Here's how the part is built. I have some questions about the finished solid (model axes, mm). Face numbers are marked on the shaded views. A direction names the side the tool comes from. Coordinates: 2 decimals unless noted, no trailing zeros. Write each loop counter-clockwise with the first axis right and the second up, starting at its lowest first coordinate (ties: lowest second). Pieces come first, ordered by that corner, then holes. Notation, with made-up numbers: (71, 36) -> (116, 36) arc R22 ccw to (116, 64) -> close; hole circle Ø6 at (-9, 43.5). An arc over 180 degrees is marked (long way). Use a Markdown table: item, result. Add a question column.
Item 1: Will these pins go through, and if not, where does the flat tip stop? pin 1 Ø2.5 at (x, y) = (-2.865, 8.89) entering from +Z; pin 2 Ø2 at (x, y) = (-5.5, -9) entering from -Z (3 decimals).
Item 2: On a 3-axis mill with a long thin cutter (end or side, diameter ignored), from which of +Z, -Z, +X, -X, +Y, -Y can I reach the whole of each face in a straight line? I mean the marked faces 4, 5 and 6. Say none if no direction works.
Item 3: If I drill on line 1 along X through (y, z) = (-9, 2.75); line 2 along Y through (x, z) = (3, 6); line 3 along X through (y, z) = (-9.5, 0.5), over which ranges is the centre line in solid material (lowest first)? Write a range as from..to.
Item 4: Imagine slicing it at B-B, the plane z = 1.75. Write out the boundary of the cut face in (x, y) (3 decimals).
Item 5: Imagine slicing it at C-C, the plane x = -7. Write out the boundary of the cut face in (y, z) (3 decimals).
Item 6: Imagine slicing it at A-A, the plane y = -8.89. Write out the boundary of the cut face in (x, z) (3 decimals), and give its area (3 significant figures).
Item 7: Imagine slicing it at D-D, the plane x = -4. Write out the boundary of the cut face in (y, z).
Item 8: If we mould it in two halves opening along Y, with no side actions, what happens to the marked faces 1, 2 and 3? For each: pulls with the +Y half, pulls with the -Y half, needs draft (parallel to the pull), parting line crosses it, or undercut.
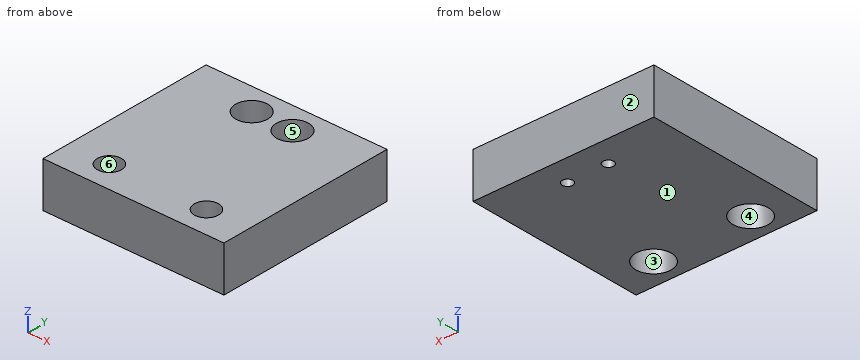
```python
from build123d import *

# Parameters (mm, degrees)
F0_W     = 25.4
F0_H     = 25.4
F0_R     = 1.7
F0_R_2   = 0.75
F1_DEPTH = 6.35
F2_R     = 2.5
F3_DEPTH = 3.175
F4_R     = 2.25
F5_DEPTH = 3.75


# Not quite as in the source:
# - a feature names something its author has since deleted; it is built from what else it names


with BuildPart() as f1:
    # F0 (on Top) → F1 (new body)
    with BuildSketch(Plane.XY):
        Rectangle(F0_W, F0_H)
        with Locations((-6.8136113696, -8.89)):
            Circle(F0_R, mode=Mode.SUBTRACT)
        with Locations((6.8136113696, -8.89)):
            Circle(F0_R, mode=Mode.SUBTRACT)
        with Locations((-2.865, 8.89)):
            Circle(F0_R_2, mode=Mode.SUBTRACT)
        with Locations((2.865, 8.89)):
            Circle(F0_R_2, mode=Mode.SUBTRACT)
    extrude(amount=F1_DEPTH)

    # F2 (on Top) → F3 (cut)
    with BuildSketch(Plane.XY):
        with Locations((-6.8136113696, -8.89)):
            Circle(F2_R)
        with Locations((6.8136113696, -8.89)):
            Circle(F2_R)
    extrude(amount=F3_DEPTH, mode=Mode.SUBTRACT)

    # F4 (on face) → F5 (cut)
    with BuildSketch(Plane.XY.offset(6.35)):
        with Locations((-2.865, 8.89)):
            Circle(F4_R)
        with Locations((2.865, 8.89)):
            Circle(F4_R)
    extrude(amount=-F5_DEPTH, mode=Mode.SUBTRACT)


solid = f1.part
```
Ans:
| question | item | result |
|---|---|---|
| 1 | pin 1 | stops at z = 2.6 |
| 1 | pin 2 | stops at z = 3.175 |
| 2 | face 4 | -Z |
| 2 | face 5 | +Z |
| 2 | face 6 | +Z, -Z |
| 3 | line 1 | x = -12.7..-9.31, -4.32..4.32, 9.31..12.7 |
| 3 | line 2 | y = -12.7..6.64, 11.14..12.7 |
| 3 | line 3 | x = -12.7..-9.24, -4.39..4.39, 9.24..12.7 |
| 4 | outline | (-12.7, -12.7) -> (12.7, -12.7) -> (12.7, 12.7) -> (-12.7, 12.7) -> close; hole circle Ø5 at (-6.814, -8.89); hole circle Ø1.5 at (-2.865, 8.89); hole circle Ø1.5 at (2.865, 8.89); hole circle Ø5 at (6.814, -8.89) |
| 5 | outline | (-12.7, 0) -> (-11.383, 0) -> (-11.383, 3.175) -> (-10.58, 3.175) -> (-10.58, 6.35) -> (-12.7, 6.35) -> close; (-7.2, 3.175) -> (-6.397, 3.175) -> (-6.397, 0) -> (12.7, 0) -> (12.7, 6.35) -> (-7.2, 6.35) -> close |
| 6 | outline | (-12.7, 0) -> (-9.314, 0) -> (-9.314, 3.175) -> (-8.514, 3.175) -> (-8.514, 6.35) -> (-12.7, 6.35) -> close; (-5.114, 3.175) -> (-4.314, 3.175) -> (-4.314, 0) -> (4.314, 0) -> (4.314, 3.175) -> (5.114, 3.175) -> (5.114, 6.35) -> (-5.114, 6.35) -> close; (8.514, 3.175) -> (9.314, 3.175) -> (9.314, 0) -> (12.7, 0) -> (12.7, 6.35) -> (8.514, 6.35) -> close |
| 6 | area | 108 mm^2 |
| 7 | outline | (-12.7, 0) -> (12.7, 0) -> (12.7, 6.35) -> (10.83, 6.35) -> (10.83, 2.6) -> (6.95, 2.6) -> (6.95, 6.35) -> (-12.7, 6.35) -> close |
| 8 | face 1 | needs draft |
| 8 | face 2 | pulls with the +Y half |
| 8 | face 3 | undercut |
